Autodesk Inventor part; units mm, degrees
ref_plane "YZ Plane" through (0, 0, 0) normal (1, 0, 0) x (0, 1, 0)
ref_plane "XZ Plane" through (0, 0, 0) normal (0, 1, 0) x (-1, 0, 0)
ref_plane "XY Plane" through (0, 0, 0) normal (0, 0, 1) x (1, 0, 0)
sketch "Sketch1" plane through (0, 0, 0) normal (0, 1, 0) x (-1, 0, 0)
  line L0 (0, 0) -> (49.2125, 0)
  line L1 (49.2125, 0) -> (49.2125, -6.35)
  line L2 (49.2125, -6.35) -> (147.6375, -6.35)
  line L3 (147.6375, -6.35) -> (147.6375, -19.05)
  line L4 (147.6375, -19.05) -> (49.2125, -19.05)
  line L5 (49.2125, -19.05) -> (49.2125, -22.225)
  line L6 (49.2125, -22.225) -> (0, -22.225)
  line L7 (0, -22.225) -> (0, 0)
  dimension "d0" = 22.225
  dimension "d1" = 147.6375
  dimension "d2" = 98.425
  dimension "d4" = 19.05
  dimension "d5" = 15.875
extrude "Extrusion1" add sketch "Sketch1" against normal blind 22.225
properties part number "Key--A"
Source: CAD feature listing. Evaluate the final solid. Frame: model axes, mm. A direction names the side the tool comes from. Round coordinates to 2 decimals unless told otherwise and drop trailing zeros. Loops run counter-clockwise (first coordinate to the right, second up) from the corner with the lowest first, then second, coordinate; pieces in that order, holes last.
Q1. Section C-C, the plane z = -1.25. Return loops of the section in (x, y) (1 decimal).
Q2. Section B-B, the plane x = -124. Return loops of the section in (y, z) (3 decimals), plus the area to 3 significant figures.
Q3. First-contact query: P1, Ø1, axis at y = -5.5, z = -20.5, coming from the -X side; P2, Ø5, axis at x = -76, y = -6.5, coming from the -Z side; P3, Ø6.5, axis at x = -107, y = -8, coming from the +Z side. Flat tips, straight axial feed; report the tip coordinate or a pass-through.
Q4. Ray query, line 1 (Z direction, x = -56, y = -10); line 2 (X direction, y = -18, z = -6). Return the intervals inside material, ascending.
Q5. Access query for faces 1 (the face through (-49.212, -11, -3)), 2 (the face through (-24, -11, 0)), 3 (the face through (-49.212, -11, -21)). Directions: +Z, -Z, +X, -X, +Y, -Y. A direction counts if a zero-diameter tool reaches every point of the face in a straight line with its end or side. Return the directions, or none.
Solutions:
1. outline: (-49.2, -22.2) - (0, -22.2) - (0, 0) - (-49.2, 0) - close
2. outline: (-22.225, -19.05) - (0, -19.05) - (0, -6.35) - (-22.225, -6.35) - close
2. area: 282 mm2
3. P1: stops at x = -49.21
3. P2: stops at z = -19.05
3. P3: stops at z = -6.35
4. line 1: z = -19.05 to -6.35
4. line 2: x = -49.21 to 0
5. face 1: +Z, -X, +Y, -Y
5. face 2: +Z, +X, -X, +Y, -Y
5. face 3: -Z, -X, +Y, -Y
